```python
from build123d import *

# Parameters (mm, degrees)
SKETCH_1_W          = 85.8
SKETCH_1_H          = 90
SKETCH_1_R          = 1.33793637
SKETCH_1_W_2        = 53.17
SKETCH_1_H_2        = 57.8
EXTRUDE_1_DEPTH     = 20
SKETCH_3_W          = 85.8
SKETCH_3_H          = 90
SKETCH_3_W_2        = 53.17
SKETCH_3_H_2        = 57.8
EXTRUDE_2_DEPTH     = 42
SKETCH_5_R          = 1.4
CUT_EXTRUDE_2_DEPTH = 20
SKETCH_5_6_W        = 65.278
SKETCH_5_6_H        = 75.438
CUT_EXTRUDE_3_DEPTH = 1.7
CUT_EXTRUDE_4_DEPTH = 28
SKETCH_8_W          = 15.4
SKETCH_8_H          = 7.281
CUT_EXTRUDE_5_DEPTH = 5
FILLET_1_R          = 2.5
FILLET_2_R          = 2.5
FILLET_3_R          = 2.5
FILLET_4_R          = 2.5
SKETCH_11_W         = 4.79539709
SKETCH_11_H         = 3.3
CUT_EXTRUDE_6_DEPTH = 10


with BuildPart() as part:
    # Sketch 1 → Extrude 1 (new body)
    with BuildSketch(Plane(origin=(0, 0, 0), x_dir=(1, 0, 0), z_dir=(0, 1, 0))):
        with Locations((38.264980184, 40.138091102)):
            Rectangle(SKETCH_1_W, SKETCH_1_H)
        with Locations(Location((1.744980184, 9.838091102, 0), (0, 0, 270))):
            Circle(SKETCH_1_R, mode=Mode.SUBTRACT)
        with Locations(Location((74.784980184, 9.838091102, 0), (0, 0, 90))):
            Circle(SKETCH_1_R, mode=Mode.SUBTRACT)
        with Locations(Location((74.784980184, 70.438091102, 0), (0, 0, 270))):
            Circle(SKETCH_1_R, mode=Mode.SUBTRACT)
        with Locations(Location((1.744980184, 70.438091102, 0), (0, 0, 90))):
            Circle(SKETCH_1_R, mode=Mode.SUBTRACT)
        with Locations((38.264980184, 40.138091102)):
            Rectangle(SKETCH_1_W_2, SKETCH_1_H_2, mode=Mode.SUBTRACT)
    extrude(amount=EXTRUDE_1_DEPTH)

    # Sketch 3 → Extrude 2 (add)
    with BuildSketch(Plane(origin=(0, 20, 0), x_dir=(1, 0, 0), z_dir=(0, 1, 0))):
        with Locations((38.264980184, 40.138091102)):
            Rectangle(SKETCH_3_W, SKETCH_3_H)
        with Locations((38.264980184, 40.138091102)):
            Rectangle(SKETCH_3_W_2, SKETCH_3_H_2, mode=Mode.SUBTRACT)
    extrude(amount=EXTRUDE_2_DEPTH)

    # Sketch 5 → Cut-Extrude 2 (cut)
    with BuildSketch(Plane(origin=(0, 62, 0), x_dir=(1, 0, 0), z_dir=(0, 1, 0))):
        with Locations(Location((7.68587004, 75.476595821, 0), (0, 0, 270))):
            Circle(SKETCH_5_R)
        with Locations(Location((68.844090328, 75.476595821, 0), (0, 0, 90))):
            Circle(SKETCH_5_R)
        with Locations(Location((68.844090328, 4.799586383, 0), (0, 0, 270))):
            Circle(SKETCH_5_R)
        with Locations(Location((7.68587004, 4.799586383, 0), (0, 0, 90))):
            Circle(SKETCH_5_R)
    extrude(amount=-CUT_EXTRUDE_2_DEPTH, mode=Mode.SUBTRACT)

    # Sketch 5_6 → Cut-Extrude 3 (cut)
    with BuildSketch(Plane(origin=(0, 62, 0), x_dir=(1, 0, 0), z_dir=(0, 1, 0))):
        with Locations((38.264980184, 40.138091102)):
            Rectangle(SKETCH_5_6_W, SKETCH_5_6_H)
    extrude(amount=-CUT_EXTRUDE_3_DEPTH, mode=Mode.SUBTRACT)

    # Sketch 7 → Cut-Extrude 4 (cut)
    with BuildSketch(Plane(origin=(0, 60.3, 0), x_dir=(1, 0, 0), z_dir=(0, 1, 0))):
        Polygon((5.625980184, 71.857091102), (11.625980184, 71.857091102), (11.625980184, 77.857091102), (64.90160291, 77.857091102), (64.90160291, 71.857091102), (70.90160291, 71.857091102), (70.903980184, 8.419091102), (64.903980184, 8.419091102), (64.903980184, 2.419091102), (11.625980184, 2.419091102), (11.625980184, 8.419091102), (5.625980184, 8.419091102), align=None)
    extrude(amount=-CUT_EXTRUDE_4_DEPTH, mode=Mode.SUBTRACT)

    # Sketch 8 → Cut-Extrude 5 (cut)
    with BuildSketch(Plane(origin=(0, 62, 0), x_dir=(1, 0, 0), z_dir=(0, 1, 0))):
        with Locations((61.997, 81.497591102)):
            Rectangle(SKETCH_8_W, SKETCH_8_H)
    extrude(amount=-CUT_EXTRUDE_5_DEPTH, mode=Mode.SUBTRACT)

    # Fillet 1
    fillet_1_edges = [part.edges().sort_by_distance(p)[0] for p in [
        (-4.635019816, 31, -85.138091102),
    ]]
    fillet(fillet_1_edges, radius=FILLET_1_R)

    # Fillet 2
    fillet_2_edges = [part.edges().sort_by_distance(p)[0] for p in [
        (81.164980184, 31, -85.138091102),
    ]]
    fillet(fillet_2_edges, radius=FILLET_2_R)

    # Fillet 3
    fillet_3_edges = [part.edges().sort_by_distance(p)[0] for p in [
        (81.164980184, 31, 4.861908898),
    ]]
    fillet(fillet_3_edges, radius=FILLET_3_R)

    # Fillet 4
    fillet_4_edges = [part.edges().sort_by_distance(p)[0] for p in [
        (-4.635019816, 31, 4.861908898),
    ]]
    fillet(fillet_4_edges, radius=FILLET_4_R)

    # Sketch 11 → Cut-Extrude 6 (cut)
    with BuildSketch(Plane(origin=(0, 0, -77.857091102), x_dir=(-1, 0, 0), z_dir=(0, 0, -1))):
        with Locations((-67.299301455, 58.65)):
            Rectangle(SKETCH_11_W, SKETCH_11_H)
    extrude(amount=-CUT_EXTRUDE_6_DEPTH, mode=Mode.SUBTRACT)


solid = part.part
```
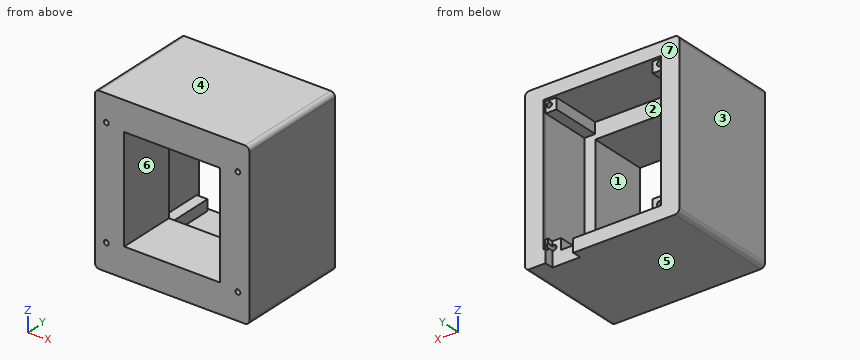
Part model, mm, in its own coordinate system. Face numbers are marked on the shaded views. A direction names the side the tool comes from. Round coordinates to 2 decimals unless told otherwise and drop trailing zeros. Loops run counter-clockwise (first coordinate to the right, second up) from the corner with the lowest first, then second, coordinate; pieces in that order, holes last. Notation, with made-up numbers: (16.25, 75.5) -> (22.25, 75.5) arc R16 cw to (22.25, 104.5) -> close; hole circle Ø10 at (-9.5, 51.25). An arc over 180 degrees is marked (long way). Use one line per item in the form item = value. Start each with the question number.
Item 1: Band-saw the part on B-B (y = 34). List the corners of the cut face in (x, z), plus the area to 3 significant figures.
Item 2: Two-plate mould, pull along Z, no slides. Class the marked faces 4, 5, 6 and 7: released by +Z, released by -Z, zero draft, split by the parting line, or undercut.
Item 3: Drill centre lines: line 1 along X through (y, z) = (36, -31); line 2 along X through (y, z) = (40, -3); line 3 along Z through (x, y) = (13, 16). Where is each one in solid material? Low to high.
Item 4: Tool access for the marked faces 1, 2 and 3: list every direction of +Z, -Z, +X, -X, +Y, -Y with a clear straight run to the whole face (end or side of a thin tool).
Item 5: Band-saw the part on D-D (y = 46.5). List the corners of the cut face in (x, z), plus the area to 3 significant figures.
Item 6: Band-saw the part on A-A (x = 60). List the corners of the cut face in (y, z).
Item 7: Drop flat-ended pins along their axis: pin 1 Ø3 at (x, z) = (66.5, -4) entering from +Y; pin 2 Ø1.3 at (x, z) = (70, -41.5) entering from +Y; pin 3 Ø1.4 at (x, z) = (8, -5) entering from +Y. Give the stop position or say it passes through.
Data:
q1.outline = (-4.64, -82.64) arc R2.5 ccw to (-2.14, -85.14) -> (78.66, -85.14) arc R2.5 ccw to (81.16, -82.64) -> (81.16, 2.36) arc R2.5 ccw to (78.66, 4.86) -> (-2.14, 4.86) arc R2.5 ccw to (-4.64, 2.36) -> close; hole (5.63, -71.86) -> (11.63, -71.86) -> (11.63, -77.86) -> (64.9, -77.86) -> (64.9, -71.86) -> (70.9, -71.86) -> (70.9, -8.42) -> (64.9, -8.42) -> (64.9, -2.42) -> (11.63, -2.42) -> (11.63, -8.42) -> (5.63, -8.42) -> close
q1.area = 2,940 mm^2
q2.face_4 = released by +Z
q2.face_5 = released by -Z
q2.face_6 = undercut
q2.face_7 = zero draft
q3.line_1 = -4.64 to 5.63, 70.9 to 81.16
q3.line_2 = -4.64 to 11.63, 64.9 to 81.16
q3.line_3 = -85.14 to -69.04, -11.24 to 4.86
q4.face_1 = +Y, -Y
q4.face_2 = +Y
q4.face_3 = +Z, -Z, -X, +Y, -Y
q5.outline = (-4.64, -82.64) arc R2.5 ccw to (-2.14, -85.14) -> (78.66, -85.14) arc R2.5 ccw to (81.16, -82.64) -> (81.16, 2.36) arc R2.5 ccw to (78.66, 4.86) -> (-2.14, 4.86) arc R2.5 ccw to (-4.64, 2.36) -> close; hole (5.63, -71.86) -> (11.63, -71.86) -> (11.63, -77.86) -> (64.9, -77.86) -> (64.9, -71.86) -> (70.9, -71.86) -> (70.9, -8.42) -> (64.9, -8.42) -> (64.9, -2.42) -> (11.63, -2.42) -> (11.63, -8.42) -> (5.63, -8.42) -> close; hole circle Ø2.8 at (7.69, -75.48); hole circle Ø2.8 at (7.69, -4.8); hole circle Ø2.8 at (68.84, -75.48); hole circle Ø2.8 at (68.84, -4.8)
q5.area = 2,910 mm^2
q6.outline = (0, -85.14) -> (57, -85.14) -> (57, -77.86) -> (32.3, -77.86) -> (32.3, -69.04) -> (0, -69.04) -> close; (0, -11.24) -> (32.3, -11.24) -> (32.3, -2.42) -> (62, -2.42) -> (62, 4.86) -> (0, 4.86) -> close
q7.pin_1 = 60.3
q7.pin_2 = 32.3
q7.pin_3 = 42
